Design review of the part shown in the three views and the two pictorial views. Dimensions are in mm from the part's minimum x, y and z. A direction names the side the tool comes from. Coordinates: 2 decimals unless noted, no trailing zeros. Loops run counter-clockwise (first coordinate to the right, second up) from the corner with the lowest first, then second, coordinate; pieces in that order, holes last. Notation, with made-up numbers: (-14, 39) -> (26, 39) arc R12 cw to (26, 62) -> close; hole circle Ø2 at (-26.5, 84.5). An arc over 180 degrees is marked (long way). One line per item, written item: value. Start each with the question number.
1. Add section C-C on z = 16. Write out the cut boundary in (x, y).
2. Add section D-D on x = 21. Write out the cut boundary in (y, z), plus the area to 3 significant figures.
3. For probe 1 along Y at (x, z) = (15, 0.9); probe 2 along Y at (x, z) = (42, 9.05); probe 3 along Z at (x, y) = (38.5, 10.5), list the stretches that pass through material, from the lowest coordinate up.
4. Insertion check: pin 1 (22 mm diameter, centred on x = 44, y = 42.5, fed in from +Z); pin 2 (14.5 mm diameter, centred on x = 45.5, z = 20.5, fed in from +Y); pin 3 (12.5 mm diameter, centred on x = 22, y = 35, fed in from +Z). Each pin has a flat end and moves straight along its axis. Give the tip position at first contact, or say it passes through.
5. Add section A-A on x = 15. Write out the cut boundary in (y, z) (3 decimals).
6. Machinability: for the marked faces 5, 6 and 7, which of the approach directions +Z, -Z, +X, -X, +Y, -Y give a long, thin tool a straight path to every point of the face, cutting with its end or side? Answer none if there is none.
7. Draft analysis for pull direction X (two halves, no side actions). For the marked faces 1, 2, 3 and 4, state which applies: pulls with the +X half, pulls with the -X half, needs draft (parallel to the pull), parting line crosses it, or undercut.
8. Add section B-B on y = 15. Write out the cut boundary in (x, z), plus the area to 3 significant figures.
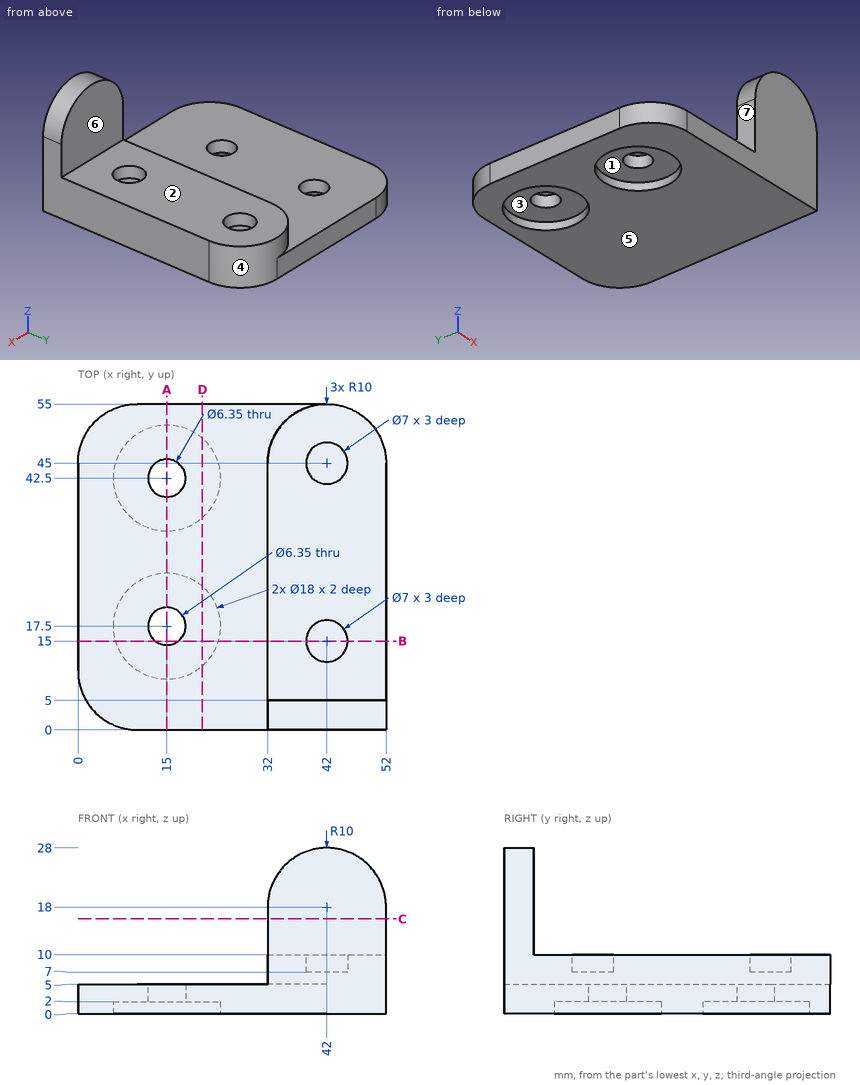
Worked answers:
1. outline: (32, 0) -> (52, 0) -> (52, 5) -> (32, 5) -> close
2. outline: (0, 0) -> (10.79, 0) -> (10.79, 2) -> (24.21, 2) -> (24.21, 0) -> (35.79, 0) -> (35.79, 2) -> (49.21, 2) -> (49.21, 0) -> (55, 0) -> (55, 5) -> (0, 5) -> close
2. area: 221 mm²
3. probe 1: y = 0 to 8.5, 26.5 to 33.5, 51.5 to 55
3. probe 2: y = 0 to 11.5, 18.5 to 41.5, 48.5 to 55
3. probe 3: z = 0 to 10
4. pin 1: stops at z = 10
4. pin 2: stops at y = 5
4. pin 3: stops at z = 5
5. outline: (0, 0) -> (8.5, 0) -> (8.5, 2) -> (14.325, 2) -> (14.325, 5) -> (0, 5) -> close; (20.675, 2) -> (26.5, 2) -> (26.5, 0) -> (33.5, 0) -> (33.5, 2) -> (39.325, 2) -> (39.325, 5) -> (20.675, 5) -> close; (45.675, 2) -> (51.5, 2) -> (51.5, 0) -> (55, 0) -> (55, 5) -> (45.675, 5) -> close
6. face 5: -Z, +X, -X, +Y, -Y
6. face 6: +Z, +X, -X, +Y
6. face 7: +Z, -X, +Y, -Y
7. face 1: undercut
7. face 2: needs draft
7. face 3: undercut
7. face 4: parting line crosses it
8. outline: (0, 0) -> (6.35, 0) -> (6.35, 2) -> (13.04, 2) -> (13.04, 5) -> (0, 5) -> close; (16.96, 2) -> (23.65, 2) -> (23.65, 0) -> (52, 0) -> (52, 10) -> (45.5, 10) -> (45.5, 7) -> (38.5, 7) -> (38.5, 10) -> (32, 10) -> (32, 5) -> (16.96, 5) -> close
8. area: 293 mm²
